Verification items for the finished model (mm, model axes). A direction names the side the tool comes from. Round coordinates to 2 decimals unless told otherwise and drop trailing zeros. Order: outer loops, then holes, each group sorted by start corner. A loop starts at its lowest first (then second) coordinate and runs counter-clockwise, first axis right, second up. Notation, with made-up numbers: (24, 16) -> (49, 16) arc R27 cw to (49, 34) -> close; hole circle Ø9 at (5, 12.25). An arc over 180 degrees is marked (long way). Return JSON: item names as keys, results as strings. Group by question number.
Item 1: Sectioned sample at A-A on y = 19. Record the cut outline in (x, z) (3 decimals).
Item 2: Draft check along X on faces 1 (the flat face through (66, 35.56, -14)), 2 (the cylindrical face through (0.2, -3.1, -15.1)), 3 (the flat face through (35.56, 14, 0)). Enter one of: pulls with the +X half, pulls with the -X half, needs draft (parallel to the pull), parting line crosses it, or undercut.
Item 3: Sectioned sample at B-B on z = 10. Record the cut outline in (x, y) (3 decimals).
Item 4: Scan lines: probe 1 along X at (y, z) = (12, -9) (3 decimals); probe 2 along X at (y, z) = (-3.25, 11.43) (3 decimals); probe 3 along Y at (x, z) = (37, 8). Record each from-to range of solid material in increasing order. Write a range as from..to.
Item 5: Access from +Z, -Z, +X, -X, +Y, -Y to the whole of each face (thin tool, end or side, straight path). Record for faces 4 (the flat face through (-35.56, 14, 0)), 5 (the flat face through (53.806, 38.215, -28.072)), 6 (the flat face through (95.623, 38, -23)), 7 (the conical face through (0.456, 39.786, -24.291)), 8 (the flat face through (0, -6.35, 0)).
Item 6: Sectioned sample at D-D on x = 39. Record the cut outline in (y, z), plus the area to 3 significant figures.
Item 7: Sectioned sample at C-C on x = -87.63. Record the cut outline in (y, z).
Item 8: Depth check by flat-ended pin: pin 1 Ø12 at (y, z) = (23, -1) entering from +X; pin 2 Ø2 at (y, z) = (31, 12) entering from -X; pin 3 Ø9.5 at (x, z) = (0, 11.43) entering from +Y. Enter the tip coordinate at first touch or a pass-through.
```python
from build123d import *

# Parameters (mm, degrees)
SKETCH1_R            = 3.675
BOSS_EXTRUDE1_DEPTH  = 6.35
BOSS_EXTRUDE2_START  = 40.64
BOSS_EXTRUDE2_DEPTH  = 40.64
CHAMFER1_SIZE        = 1.016
SKETCH3_R            = 3.2639
BOSS_EXTRUDE3_DEPTH  = 5.08
FILLET1_R            = 5.08
FILLET1_OF_MIRROR1_R = 5.08
FILLET2_R            = 1.27


with BuildPart() as part:
    # Sketch1 → Boss-Extrude1 (new body)
    with BuildSketch(Plane(origin=(0, 0, 0), x_dir=(1, 0, 0), z_dir=(0, 1, 0))):
        with BuildLine():
            Line((-35.56, 21.431101635), (-35.56, -21.431101635))
            ThreePointArc((-35.56, -21.431101635), (0, -28.575), (35.56, -21.431101635))
            Line((35.56, -21.431101635), (35.56, 21.431101635))
            ThreePointArc((35.56, 21.431101635), (0, 28.575), (-35.56, 21.431101635))
        make_face()
        with Locations(Location((-22.86, 11.43, 0), (0, 0, 270))):
            Circle(SKETCH1_R, mode=Mode.SUBTRACT)
        with Locations(Location((0, 11.43, 0), (0, 0, 270))):
            Circle(SKETCH1_R, mode=Mode.SUBTRACT)
        with Locations(Location((22.86, 11.43, 0), (0, 0, 270))):
            Circle(SKETCH1_R, mode=Mode.SUBTRACT)
        with Locations(Location((0, -11.43, 0), (0, 0, 270))):
            Circle(SKETCH1_R, mode=Mode.SUBTRACT)
    extrude(amount=-BOSS_EXTRUDE1_DEPTH)

    # Sketch2 → Boss-Extrude2 (add)
    with BuildSketch(Plane(origin=(0, 0, 0), x_dir=(1, 0, 0), z_dir=(0, 1, 0)).offset(BOSS_EXTRUDE2_START)):
        with BuildLine():
            Line((-35.56, 21.431101635), (-35.56, -21.431101635))
            ThreePointArc((-35.56, -21.431101635), (0, -28.575), (35.56, -21.431101635))
            Line((35.56, -21.431101635), (35.56, 21.431101635))
            ThreePointArc((35.56, 21.431101635), (0, 28.575), (-35.56, 21.431101635))
        make_face()
        with BuildLine():
            Line((-31.115, 18.419922333), (-31.115, -18.419922333))
            ThreePointArc((-31.115, -18.419922333), (0, -24.13), (31.115, -18.419922333))
            Line((31.115, -18.419922333), (31.115, 18.419922333))
            ThreePointArc((31.115, 18.419922333), (0, 24.13), (-31.115, 18.419922333))
        make_face(mode=Mode.SUBTRACT)
    extrude(amount=-BOSS_EXTRUDE2_DEPTH)

    # Chamfer1
    chamfer1_edges = [part.edges().sort_by_distance(p)[0] for p in [
        (0, 40.64, -24.13),
        (-31.115, 40.64, 0),
        (0, 40.64, 24.13),
        (31.115, 40.64, 0),
    ]]
    chamfer(chamfer1_edges, length=CHAMFER1_SIZE)

    # Sketch3 → Boss-Extrude3 (add)
    with BuildSketch(Plane(origin=(0, 40.64, 0), x_dir=(1, 0, 0), z_dir=(0, 1, 0))):
        Polygon((-35.56, -21.431101635), (-95.622719028, 13.246125363), (-95.622719028, 34.836125363), (-72.39, 34.836125363), (-35.56, 21.431101635), align=None)
        with Locations(Location((-87.63, 23.684417071, 0), (0, 0, 270))):
            Circle(SKETCH3_R, mode=Mode.SUBTRACT)
        with Locations(Location((-72.39, 23.684417071, 0), (0, 0, 270))):
            Circle(SKETCH3_R, mode=Mode.SUBTRACT)
        with Locations(Location((-72.39, 10.984417071, 0), (0, 0, 270))):
            Circle(SKETCH3_R, mode=Mode.SUBTRACT)
    boss_extrude3 = extrude(amount=-BOSS_EXTRUDE3_DEPTH)

    # Fillet1
    fillet1_edges = [part.edges().sort_by_distance(p)[0] for p in [
        (-95.622719028, 38.1, -13.246125363),
        (-95.622719028, 38.1, -34.836125363),
        (-72.39, 38.1, -34.836125363),
    ]]
    fillet(fillet1_edges, radius=FILLET1_R)

    # Mirror1: Boss-Extrude3 across plane
    add(boss_extrude3.mirror(Plane(origin=(0, 0, 0), x_dir=(0, 0, 1), z_dir=(1, 0, 0))))

    # Fillet1 of Mirror1
    fillet1_of_mirror1_edges = [part.edges().sort_by_distance(p)[0] for p in [
        (95.622719028, 38.1, -13.246125363),
        (95.622719028, 38.1, -34.836125363),
        (72.39, 38.1, -34.836125363),
    ]]
    fillet(fillet1_of_mirror1_edges, radius=FILLET1_OF_MIRROR1_R)

    # Fillet2
    fillet2_edges = [part.edges().sort_by_distance(p)[0] for p in [
        (35.56, 35.56, 0),
        (-35.56, 35.56, 0),
    ]]
    fillet(fillet2_edges, radius=FILLET2_R)


solid = part.part
```
Recorded:
{
 "1": {"outline": "(-35.56, -21.431) arc R92.075 ccw to (35.56, -21.431) -> (35.56, 21.431) arc R92.075 ccw to (-35.56, 21.431) -> close; hole (-31.115, -18.42) arc R87.63 ccw to (31.115, -18.42) -> (31.115, 18.42) arc R87.63 ccw to (-31.115, 18.42) -> close"},
 "2": {"face 1": "needs draft", "face 2": "undercut", "face 3": "pulls with the +X half"},
 "3": {"outline": "(-55.359, 35.56) -> (-36.83, 35.56) arc R1.27 cw to (-35.56, 34.29) -> (-35.56, -6.35) -> (-3.385, -6.35) -> (-3.385, 0) -> (-31.115, 0) -> (-31.115, 39.624) -> (-32.131, 40.64) -> (-55.359, 40.64) -> close; (3.385, -6.35) -> (35.56, -6.35) -> (35.56, 34.29) arc R1.27 cw to (36.83, 35.56) -> (55.359, 35.56) -> (55.359, 40.64) -> (32.131, 40.64) -> (31.115, 39.624) -> (31.115, 0) -> (3.385, 0) -> close"},
 "4": {"probe 1": "-35.56..-31.115, 31.115..35.56", "probe 2": "-35.56..-3.675, 3.675..35.56", "probe 3": "35.56..40.64"},
 "5": {"face 4": "+Z, -Z, -X, -Y", "face 5": "-Z, +Y, -Y", "face 6": "+Z, -Z, +X, +Y, -Y", "face 7": "+Y", "face 8": "+Z, -Z, +X, -X, -Y"},
 "6": {"outline": "(35.56, -22.68) -> (40.64, -22.68) -> (40.64, 19.45) -> (35.56, 19.45) -> close", "area": "214 mm²"},
 "7": {"outline": "(35.56, -34.84) -> (40.64, -34.84) -> (40.64, -26.95) -> (35.56, -26.95) -> close; (35.56, -20.42) -> (40.64, -20.42) -> (40.64, -8.63) -> (35.56, -8.63) -> close"},
 "8": {"pin 1": "x = 35.56", "pin 2": "x = -35.56", "pin 3": "y = 0"}
}
